Here's how the part is built. I have some questions about the finished solid (model axes, mm). Face numbers are marked on the shaded views. A direction names the side the tool comes from. Round coordinates to 2 decimals unless told otherwise and drop trailing zeros. Order: outer loops, then holes, each group sorted by start corner. A loop starts at its lowest first (then second) coordinate and runs counter-clockwise, first axis right, second up. Notation, with made-up numbers: M -16,75 L -6,75 A35 ccw -6,109 Z; hole C 13.25,26.25 d10. An arc over 180 degrees is marked long. Use one line per item in the form item = value. Start each with the question number.
Autodesk Inventor part; units mm, degrees
ref_plane "YZ Plane" through (0, 0, 0) normal (1, 0, 0) x (0, 1, 0)
ref_plane "XZ Plane" through (0, 0, 0) normal (0, 1, 0) x (-1, 0, 0)
ref_plane "XY Plane" through (0, 0, 0) normal (0, 0, 1) x (1, 0, 0)
sketch "Szkic1" plane through (0, 0, 0) normal (0, 0, 1) x (1, 0, 0)
  circle A0 centre (0, 0) radius 9.5
  circle A1 centre (0, 0) radius 3.185
  dimension "d0" = 19
  dimension "d3" = 6.37
extrude "Wyciągnięcie proste2" add sketch "Szkic1" along normal blind 6
sketch "Szkic2" plane through (0, 0, 6) normal (0, 0, 1) x (1, 0, 0)
  circle A0 centre (0, 0) radius 3.185
  circle A1 centre (0, 0) radius 16
  circle A2 centre (0, 0) radius 3.185
  dimension "d6" = 32
extrude "Wyciągnięcie proste3" add sketch "Szkic2" along normal blind 2
sketch "Szkic3" plane through (0, 0, 8) normal (0, 0, 1) x (1, 0, 0)
  circle A0 centre (0, 0) radius 8
  circle A1 centre (0, 0) radius 3.185
  line L0 (0, 8) -> (0, 11) construction
  line L1 (-0.5, 11) -> (0.5, 11)
  line L2 (0.5, 11) -> (1.1475, 7.9173)
  line L3 (-0.5, 11) -> (-1.1475, 7.9173)
  line L4 (-3.2539, 7.3084) -> (-4.4741, 10.049) construction
  line L5 (-4.9309, 9.8456) -> (-4.2686, 6.766)
  line L6 (-4.9309, 9.8456) -> (-4.0173, 10.2524)
  line L7 (-4.0173, 10.2524) -> (-2.1719, 7.6995)
  line L8 (-5.9452, 5.353) -> (-8.1746, 7.3604) construction
  line L9 (-8.5092, 6.9889) -> (-6.6515, 4.4449)
  line L10 (-8.5092, 6.9889) -> (-7.84, 7.732)
  line L11 (-7.84, 7.732) -> (-5.1158, 6.1505)
  line L12 (-7.6085, 2.4721) -> (-10.4616, 3.3992) construction
  line L13 (-10.6161, 2.9237) -> (-7.8844, 1.3552)
  line L14 (-10.6161, 2.9237) -> (-10.3071, 3.8747)
  line L15 (-10.3071, 3.8747) -> (-7.1752, 3.5379)
  line L16 (-7.9562, -0.8362) -> (-10.9397, -1.1498) construction
  line L17 (-10.8875, -1.6471) -> (-7.754, -1.9688)
  line L18 (-10.8875, -1.6471) -> (-10.992, -0.6526)
  line L19 (-10.992, -0.6526) -> (-7.9938, 0.3137)
  line L20 (-6.9282, -4) -> (-9.5263, -5.5) construction
  line L21 (-9.2763, -5.933) -> (-6.2828, -4.9524)
  line L22 (-9.2763, -5.933) -> (-9.7763, -5.067)
  line L23 (-9.7763, -5.067) -> (-7.4303, -2.9649)
  line L24 (-4.7023, -6.4721) -> (-6.4656, -8.8992) construction
  line L25 (-6.0611, -9.1931) -> (-3.7253, -7.0797)
  line L26 (-6.0611, -9.1931) -> (-6.8701, -8.6053)
  line L27 (-6.8701, -8.6053) -> (-5.582, -5.7307)
  line L28 (-1.6633, -7.8252) -> (-2.287, -10.7596) construction
  line L29 (-1.798, -10.8636) -> (-0.5236, -7.9828)
  line L30 (-1.798, -10.8636) -> (-2.7761, -10.6557)
  line L31 (-2.7761, -10.6557) -> (-2.7685, -7.5057)
  line L32 (1.6633, -7.8252) -> (2.287, -10.7596) construction
  line L33 (2.7761, -10.6557) -> (2.7685, -7.5057)
  line L34 (2.7761, -10.6557) -> (1.798, -10.8636)
  line L35 (1.798, -10.8636) -> (0.5236, -7.9828)
  line L36 (4.7023, -6.4721) -> (6.4656, -8.8992) construction
  line L37 (6.8701, -8.6053) -> (5.582, -5.7307)
  line L38 (6.8701, -8.6053) -> (6.0611, -9.1931)
  line L39 (6.0611, -9.1931) -> (3.7253, -7.0797)
  line L40 (6.9282, -4) -> (9.5263, -5.5) construction
  line L41 (9.7763, -5.067) -> (7.4303, -2.9649)
  line L42 (9.7763, -5.067) -> (9.2763, -5.933)
  line L43 (9.2763, -5.933) -> (6.2828, -4.9524)
  line L44 (7.9562, -0.8362) -> (10.9397, -1.1498) construction
  line L45 (10.992, -0.6526) -> (7.9938, 0.3137)
  line L46 (10.992, -0.6526) -> (10.8875, -1.6471)
  line L47 (10.8875, -1.6471) -> (7.754, -1.9688)
  line L48 (7.6085, 2.4721) -> (10.4616, 3.3992) construction
  line L49 (10.3071, 3.8747) -> (7.1752, 3.5379)
  line L50 (10.3071, 3.8747) -> (10.6161, 2.9237)
  line L51 (10.6161, 2.9237) -> (7.8844, 1.3552)
  line L52 (5.9452, 5.353) -> (8.1746, 7.3604) construction
  line L53 (7.84, 7.732) -> (5.1158, 6.1505)
  line L54 (7.84, 7.732) -> (8.5092, 6.9889)
  line L55 (8.5092, 6.9889) -> (6.6515, 4.4449)
  line L56 (3.2539, 7.3084) -> (4.4741, 10.049) construction
  line L57 (4.0173, 10.2524) -> (2.1719, 7.6995)
  line L58 (4.0173, 10.2524) -> (4.9309, 9.8456)
  line L59 (4.9309, 9.8456) -> (4.2686, 6.766)
  dimension "d9" = 16
  dimension "d10" = 3
  dimension "d11" = 1
  dimension "d12" = 3.15
  dimension "d15" = 360
extrude "Wyciągnięcie proste4" add sketch "Szkic3" along normal blind 11
sketch "Szkic4" plane through (0, 0, 19) normal (0, 0, 1) x (1, 0, 0)
  point P0 (0, 0)
fillet "Zaokrąglenie1" radius 0.5 1 edges at (-16, 0, 8)
fillet "Zaokrąglenie2" radius 0.5 4 edges at (-16, 0, 6) (-9.5, 0, 0) (-3.185, 0, 19) (-3.185, 0, 0)
properties part number "kolo_zebate_do_pasa_fi32_6,370_L19"
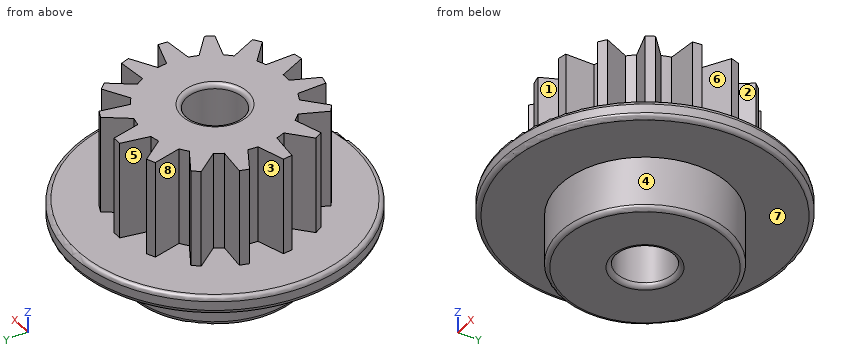
1) On a 3-axis mill with a long thin cutter (end or side, diameter ignored), from which of +Z, -Z, +X, -X, +Y, -Y can I reach the whole of each face in a straight line? I mean the marked faces 1, 2, 3, 4 and 5. Say none if no direction works.
2) If I drill on line 1 (Y direction, x = 0, z = 15) (3 decimals); line 2 (Y direction, x = 0, z = 4.5) (3 decimals); line 3 (Z direction, x = 9, y = 11), over which ranges is the centre line in solid material (lowest first)?
3) Will these pins go through, and if not, where does the flat tip stop? pin 1 Ø1 at (y, z) = (8, 12) entering from -X; pin 2 Ø4 at (y, z) = (-8.5, 16) entering from +X; pin 3 Ø6 at (x, z) = (-9, 5.5) entering from +Y; pin 4 Ø8.5 at (x, y) = (0, 0) entering from +Z.
4) If we section it at A-A on x = 0: Write out the boundary of the cut face in (y, z) (3 decimals), then the cut area to 3 significant figures.
5) If we section it at B-B on z = 5.25: Write out the boundary of the cut face in (x, y) (3 decimals).
6) If we mould it in two halves opening along X, with no side actions, what happens to the marked faces 6, 7 and 8? For each: +X half, -X half, draft (parallel to the pull), parting line (faces both ways), or undercut.
Completed:
q1.face_1 = +Z, -Y
q1.face_2 = +Z, +X
q1.face_3 = +Z, -X
q1.face_4 = -Z
q1.face_5 = +Z, +Y
q2.line_1 = -8 to -3.185, 3.185 to 11
q2.line_2 = -9.5 to -3.185, 3.185 to 9.5
q2.line_3 = 6 to 8
q3.pin_1 = -8.05
q3.pin_2 = 6.87
q3.pin_3 = 14.77
q3.pin_4 = 19
q4.outline = M -16,6.5 A0.5 ccw -15.5,6 L -9.5,6 L -9.5,0.5 A0.5 ccw -9,0 L -3.685,0 A0.5 ccw -3.185,0.5 L -3.185,18.5 A0.5 ccw -3.685,19 L -8,19 L -8,8 L -15.5,8 A0.5 ccw -16,7.5 Z; M 3.185,0.5 A0.5 ccw 3.685,0 L 9,0 A0.5 ccw 9.5,0.5 L 9.5,6 L 15.5,6 A0.5 ccw 16,6.5 L 16,7.5 A0.5 ccw 15.5,8 L 11,8 L 11,19 L 3.685,19 A0.5 ccw 3.185,18.5 Z
q4.area = 265 mm²
q5.outline = C 0,0 d19; hole C 0,0 d6.37
q6.face_6 = +X half
q6.face_7 = draft
q6.face_8 = undercut
